```python
from build123d import *

# Parameters (mm, degrees)
SKETCH1_W           = 12.7
SKETCH1_H           = 3.175
BOSS_EXTRUDE1_DEPTH = 69.85
SKETCH2_W           = 12.7
SKETCH2_H           = 3.175
BOSS_EXTRUDE2_DEPTH = 19.05
SKETCH3_R           = 1.27
CUT_EXTRUDE1_DEPTH  = 71.084124673
SKETCH4_R           = 1.27
CUT_EXTRUDE2_DEPTH  = 73.679071953
CUT_EXTRUDE3_DEPTH  = 73.679071953


with BuildPart() as part:
    # Sketch1 → Boss-Extrude1 (new body)
    with BuildSketch(Plane(origin=(0, 0, 0), x_dir=(1, 0, 0), z_dir=(0, 1, 0))):
        Rectangle(SKETCH1_W, SKETCH1_H)
    extrude(amount=BOSS_EXTRUDE1_DEPTH)

    # Sketch2 → Boss-Extrude2 (add)
    with BuildSketch(Plane.XY.offset(1.5875)):
        with Locations((0, 68.2625)):
            Rectangle(SKETCH2_W, SKETCH2_H)
    extrude(amount=BOSS_EXTRUDE2_DEPTH)

    # Sketch3 → Cut-Extrude1 (cut, through all)
    with BuildSketch(Plane.XZ.offset(-66.675)):
        with Locations(Location((0, 17.4625, 0), (0, 0, 270))):
            Circle(SKETCH3_R)
    extrude(amount=-CUT_EXTRUDE1_DEPTH, mode=Mode.SUBTRACT)

    # Sketch4 → Cut-Extrude2 (cut, through all)
    with BuildSketch(Plane.XY.offset(1.5875)):
        with Locations((0, 21.59)):
            Circle(SKETCH4_R)
        with Locations((0, 60.325)):
            Circle(SKETCH4_R)
    extrude(amount=-CUT_EXTRUDE2_DEPTH, mode=Mode.SUBTRACT)

    # Sketch6 → Cut-Extrude3 (cut, through all)
    with BuildSketch(Plane.XY.offset(1.5875)):
        Polygon((3.951482723, 0), (6.35, 5.27166953), (6.35, 0), align=None)
    extrude(amount=-CUT_EXTRUDE3_DEPTH, mode=Mode.SUBTRACT)


solid = part.part
```
Source: CAD feature listing. Evaluate the final solid. Frame: model axes, mm. A direction names the side the tool comes from. Give positions to 0.01 mm unless a question says otherwise; leave off trailing zeros. Order: outer loops, then holes, each group sorted by start corner. A loop starts at its lowest first (then second) coordinate and runs counter-clockwise, first axis right, second up.
(1) Pull-direction query (Z, two-part tool) for faces 1 (the face through (0.06, 68.24, 18.73)), 2 (the face through (-1, 0, 0)), 3 (the face through (0, 34, -1.588)); classes: +Z half, -Z half, draft (parallel to the pull), parting line (faces both ways), or undercut.
(2) Section query A-A (y = 21.59). Return the cut outline in (x, z).
(3) Section query B-B (x = 0). State how many separate pieces and enclosed holes the cut face has, plus the area to 3 significant figures.
(4) Access query for faces 4 (the face through (0, 66.675, 11)), 5 (the face through (0, 68, 20.638)). Directions: +Z, -Z, +X, -X, +Y, -Y. A direction counts if a zero-diameter tool reaches every point of the face in a straight line with its end or side. Return the directions, or none.
(5) Section query C-C (z = 10.5). Return the cut outline in (x, y) (3 decimals), plus the area to 3 significant figures.
(6) Material intervals for line 1 along Y through (x, z) = (0, 0.15) (3 decimals); line 2 along Y through (x, z) = (-0.25, -0.5); line 3 along Z through (x, y) = (4.5, 53), sorted ascending.
(7) Contact query for flat-ended pins moving along their axis: P1, Ø6.5, axis at x = 0, z = 9, coming from the -Y side (3 decimals); P2, Ø10, axis at y = 46, z = 7, coming from the -X side; P3, Ø3.5, axis at x = 0, y = 60.325, coming from the -Z side; P4, Ø4, axis at x = -3, y = 42.5, coming from the +Z side. Output: stop coordinate, or through.
Outcome:
1. face 1: undercut
1. face 2: draft
1. face 3: -Z half
2. outline: (-6.35, -1.59) - (-1.27, -1.59) - (-1.27, 1.59) - (-6.35, 1.59) - close; (1.27, -1.59) - (6.35, -1.59) - (6.35, 1.59) - (1.27, 1.59) - close
3. separate pieces: 4
3. enclosed holes: 0
3. area: 258 mm2
4. face 4: +Z, +X, -X, -Y
4. face 5: +Z, +X, -X, +Y, -Y
5. outline: (-6.35, 66.675) - (6.35, 66.675) - (6.35, 69.85) - (-6.35, 69.85) - close
5. area: 40.3 mm2
6. line 1: y = 0 to 20.32, 22.86 to 59.055, 61.595 to 69.85
6. line 2: y = 0 to 20.34, 22.84 to 59.08, 61.57 to 69.85
6. line 3: z = -1.59 to 1.59
7. P1: stops at y = 66.675
7. P2: passes through
7. P3: stops at z = -1.59
7. P4: stops at z = 1.59
